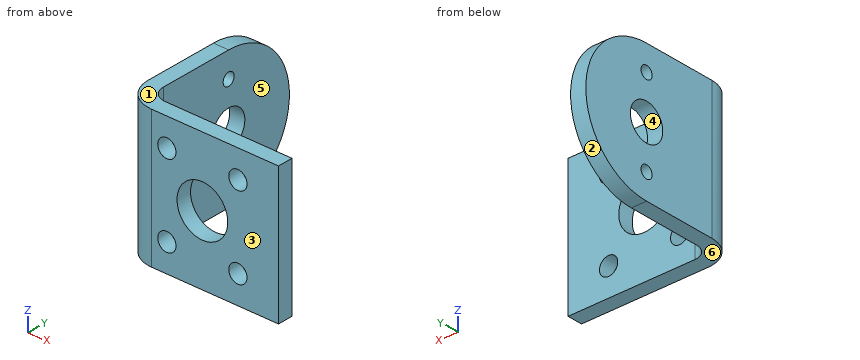
Autodesk Inventor part; units mm, degrees
ref_plane "YZ Plane" through (0, 0, 0) normal (1, 0, 0) x (0, 1, 0)
ref_plane "XZ Plane" through (0, 0, 0) normal (0, 1, 0) x (-1, 0, 0)
ref_plane "XY Plane" through (0, 0, 0) normal (0, 0, 1) x (1, 0, 0)
sketch "草图1" plane through (0, 0, 0) normal (0, 0, 1) x (1, 0, 0)
  line L0 (-16.146, 12.8249) -> (-13.146, 12.8249)
  line L1 (-13.146, 12.8249) -> (-13.146, -15.1751)
  line L2 (-16.146, -15.1751) -> (-16.146, 12.8249)
  arc A0 (-13.146, -15.1751) -> (-10.146, -18.1751) centre (-10.146, -15.1751) ccw
  line L3 (-10.146, -18.1751) -> (-10.146, -15.1751) construction
  arc A1 (-16.146, -15.1751) -> (-10.146, -21.1751) centre (-10.146, -15.1751) ccw
  line L4 (-10.146, -18.1751) -> (14.854, -18.1751)
  line L5 (-10.146, -21.1751) -> (14.854, -21.1751)
  line L6 (14.854, -18.1751) -> (14.854, -21.1751)
  point P0 (0, 0)
  dimension "d0" = 3
  dimension "d1" = 28
  dimension "d2" = 28
  dimension "d3" = 3
  dimension "d4" = 25
  dimension "d5" = 25
extrude "拉伸1" add sketch "草图1" along normal blind 27
sketch "草图2" plane through (-16.146, -15.1751, 0) normal (-1, 0, 0) x (0, 0, 1)
  line L0 (0, 28) -> (0, 0) construction
  line L1 (27, 0) -> (27, -3) construction
  line L2 (0, 28) -> (27, 28) construction
  line L3 (27, 28) -> (27, 0) construction
  line L4 (27, 0) -> (0, 0) construction
  line L5 (0, 0) -> (0, 28) construction
  line L6 (0, 14.5) -> (27, 14.5) construction
  line L7 (27, 0) -> (27, 28) construction
  point P0 (0, 15.1751)
  dimension "d8" = 13.5
sketch "草图3" plane through (-13.146, -15.1751, 0) normal (1, 0, 0) x (0, 0, -1)
  line L0 (-27, 0) -> (-27, 28) construction
  line L1 (0, 0) -> (0, -3) construction
  line L2 (-27, 28) -> (0, 28) construction
  line L3 (0, 28) -> (0, 0) construction
  line L4 (0, 0) -> (-27, 0) construction
  line L5 (-27, 0) -> (-27, 28) construction
  line L6 (-27, 14.5) -> (0, 14.5) construction
  line L7 (0, 28) -> (-27, 28) construction
  arc A0 (0, 14.5) -> (-27, 14.5) centre (-13.5, 14.5) ccw
  line L8 (-27, 14.5) -> (-27, 28)
  line L9 (-13.5, 28) -> (-27, 28)
  line L10 (-13.5, 28) -> (0, 28)
  line L11 (0, 28) -> (0, 0)
  line L12 (0, 14.5) -> (0, 28)
  circle A1 centre (-13.5, 14.5) radius 3.6
  circle A2 centre (-5, 14.5) radius 1.23
  line L13 (-13.5, 14.5) -> (-13.5, 0) construction
  circle A3 centre (-22, 14.5) radius 1.23
  point P0 (0, 15.1751)
  dimension "d9" = 13.5
  dimension "d12" = 7.2
  dimension "d13" = 2.46
  dimension "d14" = 17
extrude "拉伸2" cut sketch "草图3" against normal through all contours A0 L8 L9 | A0 L10 L11
extrude "拉伸3" cut sketch "草图3" against normal through all contours A1 | A2 | A3
sketch "草图4" plane through (-10.146, -18.1751, 0) normal (0, 1, 0) x (1, 0, 0)
  point P0 (10.146, 0)
sketch "草图5" plane through (-10.146, -18.1751, 0) normal (0, 1, 0) x (1, 0, 0)
  circle A0 centre (10, -13.5) radius 5
  line L0 (25, 0) -> (0, 0)
  line L1 (25, 0) -> (25, -27)
  line L2 (10, -13.5) -> (10, -3.684) construction
  line L3 (10, -13.5) -> (-1.3209, -13.5) construction
  point P0 (10.146, 0)
  point P1 (3, -5.5)
  point P2 (3, -21.5)
  point P3 (17, -5.5)
  point P4 (17, -21.5)
  dimension "d17" = 10
  dimension "d18" = 13.5
  dimension "d19" = 15
  dimension "d20" = 16
  dimension "d21" = 14
  dimension "d22" = 7
  dimension "d23" = 7
extrude "拉伸4" cut sketch "草图5" against normal through all
hole "孔1" at (-7.146, -18.1751, 21.5) at (-7.146, -18.1751, 5.5) at (6.854, -18.1751, 5.5) at (6.854, -18.1751, 21.5) direction (0, -1, 0) diameter 3.6 end through all
properties part number "联轴器"
Model file for the job. Use its own axes, mm. Face numbers are marked on the shaded views. A direction names the side the tool comes from. Coordinates: 2 decimals unless noted, no trailing zeros. Loops run counter-clockwise (first coordinate to the right, second up) from the corner with the lowest first, then second, coordinate; pieces in that order, holes last. Notation, with made-up numbers: M 47.5,57.5 L 78.5,57.5 A28 ccw 78.5,75.5 Z; hole C 81.5,79 d5. An arc over 180 degrees is marked long. Use CSV: the item, a comma, the result in double quotes. Start each with the question number.
1. Probe probe 1 along X at (y, z) = (-19.3, 21.5); probe 2 along X at (y, z) = (-19.2, 5.5); probe 3 along X at (y, z) = (5, 23.75). List the from-to ranges inside material, lowest first. Write a range as [from, to].
2. Band-saw the part on C-C, the plane x = 0.5. List the corners of the cut face in (y, z), then the cut area to 3 significant figures.
3. Two-plate mould, pull along Z, no slides. Class the marked faces 1, 2, 3 and 4: pulls with the +Z half, pulls with the -Z half, needs draft (parallel to the pull), parting line crosses it, or undercut.
4. Band-saw the part on A-A, the plane z = 13.5. List the corners of the cut face in (x, y).
5. Flat gauge pins, fed straight in: pin 1 (4 mm diameter, centred on y = -0.68, z = 5, fed in from +X); pin 2 (13 mm diameter, centred on x = -0.146, z = 13.5, fed in from +Y); pin 3 (4.5 mm diameter, centred on y = -0.68, z = 13.5, fed in from -X). Where does each tip first touch, or does it go through?
6. Tool access for the marked faces 5 and 6: list every direction of +Z, -Z, +X, -X, +Y, -Y with a clear straight run to the whole face (end or side of a thin tool).
7. Band-saw the part on B-B, the plane z = 22. List the corners of the cut face in (x, y), then the cut area to 3 significant figures.
8. Band-saw the part on D-D, the plane z = 9.25. List the corners of the cut face in (x, y), then the cut area to 3 significant figures.
Entries:
1,probe 1,"x = [-14.5, -8.95], [-5.35, 5.05], [8.65, 14.85]"
1,probe 2,"x = [-14.6, -8.95], [-5.35, 5.05], [8.65, 14.85]"
1,probe 3,"x = [-16.15, -13.15]"
2,outline,"M -21.18,0 L -18.18,0 L -18.18,8.54 L -21.18,8.54 Z; M -21.18,18.46 L -18.18,18.46 L -18.18,27 L -21.18,27 Z"
2,area,"51.3 mm2"
3,face 1,"pulls with the +Z half"
3,face 2,"parting line crosses it"
3,face 3,"needs draft"
3,face 4,"undercut"
4,outline,"M -16.15,-15.18 A6 ccw -10.15,-21.18 L -5.15,-21.18 L -5.15,-18.18 L -10.15,-18.18 A3 cw -13.15,-15.18 L -13.15,-4.28 L -16.15,-4.28 Z; M -16.15,2.92 L -13.15,2.92 L -13.15,12.82 L -16.15,12.82 Z; M 4.85,-21.18 L 14.85,-21.18 L 14.85,-18.18 L 4.85,-18.18 Z"
5,pin 1,"stops at x = -13.15"
5,pin 2,"stops at y = -18.18"
5,pin 3,"passes through"
6,face 5,"+Z, -Z, +X, +Y"
6,face 6,"-Z, +X, -X, +Y, -Y"
7,outline,"M -16.15,-15.18 A6 ccw -10.15,-21.18 L -8.88,-21.18 L -8.88,-18.18 L -10.15,-18.18 A3 cw -13.15,-15.18 L -13.15,-1.91 L -16.15,-1.91 Z; M -16.15,0.55 L -13.15,0.55 L -13.15,9.81 L -16.15,9.81 Z; M -5.42,-21.18 L 5.12,-21.18 L 5.12,-18.18 L -5.42,-18.18 Z; M 8.58,-21.18 L 14.85,-21.18 L 14.85,-18.18 L 8.58,-18.18 Z"
7,area,"143 mm2"
8,outline,"M -16.15,-15.18 A6 ccw -10.15,-21.18 L -2.78,-21.18 L -2.78,-18.18 L -10.15,-18.18 A3 cw -13.15,-15.18 L -13.15,12.14 L -16.15,12.14 Z; M 2.49,-21.18 L 14.85,-21.18 L 14.85,-18.18 L 2.49,-18.18 Z"
8,area,"162 mm2"
